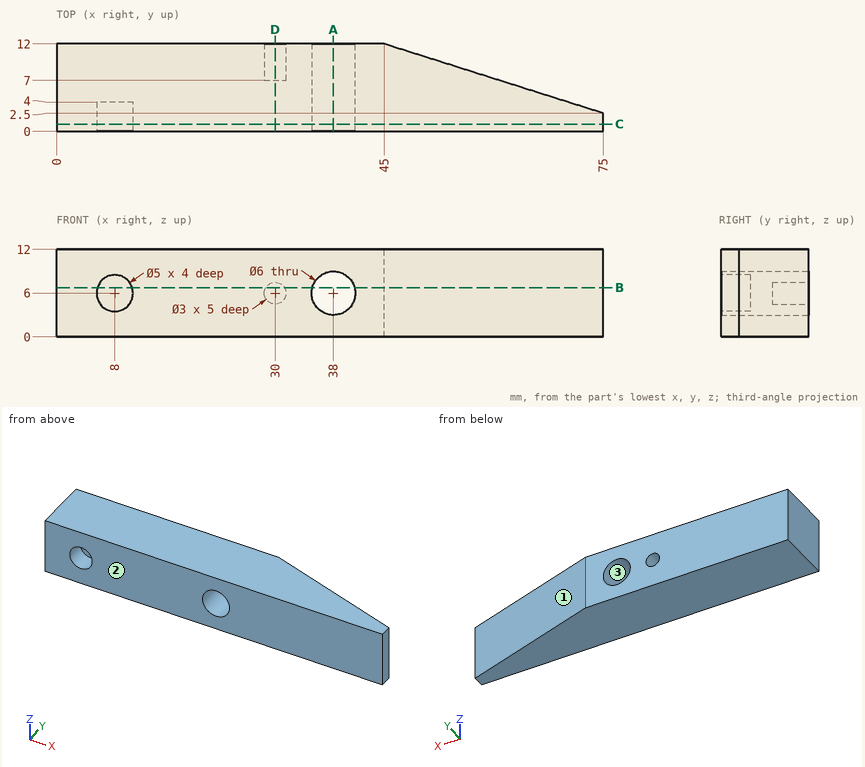
Here's the drawing with two shaded views (mm, measured from the low corner). I have some questions. Give positions to 0.01 mm unless a question says otherwise; leave off trailing zeros. Loops run counter-clockwise (first coordinate to the right, second up) from the corner with the lowest first, then second, coordinate; pieces in that order, holes last. Notation, with made-up numbers: (67.25, -25.75) - (83.25, -25.75) arc R29 cw to (83.25, -0.75) - close; hole circle Ø11 at (23.5, 11). An arc over 180 degrees is marked (long way). Answer in a Markdown table with one row per item. Add a question column.
Q1. For pin 1 (5.5 mm diameter, centred on x = 38, z = 6, fed in from +Y); pin 2 (1.8 mm diameter, centred on x = 30, z = 6, fed in from +Y), each with a flat end and sliding along its axis, tell me the tip position at first contact or that it passes through.
Q2. If we section it at B-B (z = 6.75): List the corners of the cut face in (x, y) for me, plus the area to 3 significant figures.
Q3. Please list where these lines run through material, in increasing order: L1, parallel to Z at x = 8, y = 1.5; L2, parallel to Z at x = 38, y = 9; L3, parallel to Y at x = 30, z = 7. Write a range as from..to.
Q4. If we section it at A-A (x = 38): List the corners of the cut face in (y, z) for me, plus the area to 3 significant figures.
Q5. If we section it at C-C (y = 1): List the corners of the cut face in (x, z) for me, plus the area to 3 significant figures.
Q6. If we section it at D-D (x = 30): List the corners of the cut face in (y, z) for me, plus the area to 3 significant figures.
Q7. We'd pull the mould along X, two halves only. Please class the marked faces 1, 2 and 3: +X half, -X half, draft (parallel to the pull), parting line (faces both ways), or undercut.
The answers:
| question | item | result |
|---|---|---|
| 1 | pin 1 | passes through |
| 1 | pin 2 | stops at y = 7 |
| 2 | outline | (0, 0) - (5.62, 0) - (5.62, 4) - (10.38, 4) - (10.38, 0) - (35.1, 0) - (35.1, 12) - (31.3, 12) - (31.3, 7) - (28.7, 7) - (28.7, 12) - (0, 12) - close; (40.9, 0) - (75, 0) - (75, 2.5) - (45, 12) - (40.9, 12) - close |
| 2 | area | 656 mm^2 |
| 3 | L1 | z = 0..3.5, 8.5..12 |
| 3 | L2 | z = 0..3, 9..12 |
| 3 | L3 | y = 0..7 |
| 4 | outline | (0, 0) - (12, 0) - (12, 3) - (0, 3) - close; (0, 9) - (12, 9) - (12, 12) - (0, 12) - close |
| 4 | area | 72.0 mm^2 |
| 5 | outline | (0, 0) - (75, 0) - (75, 12) - (0, 12) - close; hole circle Ø5 at (8, 6); hole circle Ø6 at (38, 6) |
| 5 | area | 852 mm^2 |
| 6 | outline | (0, 0) - (12, 0) - (12, 4.5) - (7, 4.5) - (7, 7.5) - (12, 7.5) - (12, 12) - (0, 12) - close |
| 6 | area | 129 mm^2 |
| 7 | face 1 | +X half |
| 7 | face 2 | draft |
| 7 | face 3 | undercut |
